For this review, take the finished solid that the model builds, in its own axes (mm). A direction names the side the tool comes from. Give positions to 0.01 mm unless a question says otherwise; leave off trailing zeros. Loops run counter-clockwise (first coordinate to the right, second up) from the corner with the lowest first, then second, coordinate; pieces in that order, holes last. Notation, with made-up numbers: (16, 38) -> (36, 38) arc R22 cw to (36, 71) -> close; hole circle Ø8 at (-33.5, -27.75). An arc over 180 degrees is marked (long way). Answer as CSV lines item,"result". Start each with the question number.
Item 1: Machinability: for faces 1 (the face through (0.445, -20.414, -23.491)), 2 (the face through (-13.1, 53.9, -1.2)), which of the approach directions +Z, -Z, +X, -X, +Y, -Y give a long, thin tool a straight path to every point of the face, cutting with its end or side? Answer none if there is none.
Item 2: Add section A-A on x = 0. State how many separate pieces and enclosed holes the cut face has, plus the area to 3 significant figures.
Item 3: Clearance check with a flat-ended pin moving along its axis: P1, Ø17, axis at x = 0, y = -6.35, coming from the +Z side. State where the tip first meets the part, or that it passes through.
Item 4: The part is to be moulded in two halves that separate along X. For faces 3 (the face through (36.191, 58.514, -0.267)), 4 (the face through (0, 20, -25.4)), 5 (the face through (-2.06, -15.65, -0.36)), say which applies: +X half, -X half, draft (parallel to the pull), parting line (faces both ways), or undercut.
Item 5: For L1, parallel to Z at x = -7, y = 44; L2, parallel to Y at x = -5.5, z = -5 (3 decimals); L3, parallel to Y at x = 7, z = 2.5 (3 decimals), list the stretches that pass through material, from the lowest coordinate up. Write a range as from..to.
Item 6: Add section D-D on y = 44.45. State the section outline as (x, z) points (3 decimals).
Item 7: Add section B-B on y = -6.35. State the section outline as (x, z) points (3 decimals), plus the area to 3 significant figures.
```python
from build123d import *

# Parameters (mm, degrees)
SKETCH1_W           = 76.2
SKETCH1_H           = 82.55
SKETCH1_R           = 9.525
BOSS_EXTRUDE1_DEPTH = 25.4
SKETCH2_R           = 9.525
CUT_EXTRUDE1_DEPTH  = 50.8
FILLET1_R           = 6.35


with BuildPart() as part:
    # Sketch1 → Boss-Extrude1 (new, symmetric)
    with BuildSketch(Plane.XY):
        with Locations((0, 19.05)):
            Rectangle(SKETCH1_W, SKETCH1_H)
        with Locations((0, -6.35)):
            Circle(SKETCH1_R, mode=Mode.SUBTRACT)
    extrude(amount=BOSS_EXTRUDE1_DEPTH, both=True)

    # Sketch2 → Cut-Extrude1 (cut)
    with BuildSketch(Plane.ZY.offset(38.1)):
        with Locations((0, 44.45)):
            Circle(SKETCH2_R)
    extrude(amount=-CUT_EXTRUDE1_DEPTH, mode=Mode.SUBTRACT)

    # Fillet1
    fillet1_edges = [part.edges().sort_by_distance(p)[0] for p in [
        (-38.1, 19.05, 25.4),
        (0, -22.225, 25.4),
        (38.1, 19.05, 25.4),
        (0, -22.225, -25.4),
        (-38.1, 19.05, -25.4),
        (0, 60.325, -25.4),
        (38.1, 19.05, -25.4),
        (38.1, -22.225, 0),
        (-38.1, -22.225, 0),
        (-38.1, 60.325, 0),
        (38.1, 60.325, 0),
        (0, 60.325, 25.4),
    ]]
    fillet(fillet1_edges, radius=FILLET1_R - 0.0001)  # a hair under: the kernel refuses the full size


solid = part.part
```
Computed values:
1,face 1,"-Z, +X, -X, -Y"
1,face 2,"-X"
2,separate pieces,"2"
2,enclosed holes,"1"
2,area,"2,910 mm²"
3,P1,"through"
4,face 3,"+X half"
4,face 4,"draft"
4,face 5,"undercut"
5,L1,"-25.4..-9.51, 9.51..25.4"
5,L2,"-22.225..-14.127, 1.427..36.343, 52.557..60.325"
5,L3,"-22.225..-12.81, 0.11..35.259, 53.641..60.325"
6,outline,"(-38.1, -19.05) arc R6.35 ccw to (-31.75, -25.4) -> (31.75, -25.4) arc R6.35 ccw to (38.1, -19.05) -> (38.1, 19.05) arc R6.35 ccw to (31.75, 25.4) -> (-31.75, 25.4) arc R6.35 ccw to (-38.1, 19.05) -> (-38.1, 9.525) -> (12.7, 9.525) -> (12.7, -9.525) -> (-38.1, -9.525) -> close"
7,outline,"(-38.1, -19.05) arc R6.35 ccw to (-31.75, -25.4) -> (-9.525, -25.4) -> (-9.525, 25.4) -> (-31.75, 25.4) arc R6.35 ccw to (-38.1, 19.05) -> close; (9.525, -25.4) -> (31.75, -25.4) arc R6.35 ccw to (38.1, -19.05) -> (38.1, 19.05) arc R6.35 ccw to (31.75, 25.4) -> (9.525, 25.4) -> close"
7,area,"2,870 mm²"
